from build123d import *

# Parameters (mm, degrees)
CROQUIS1_W              = 1660
CROQUIS1_H              = 810
CROQUIS1_W_2            = 300
CROQUIS1_H_2            = 5
SALIENTE_EXTRUIR3_DEPTH = 5
CROQUIS2_W              = 5
CROQUIS2_H              = 40
CROQUIS2_W_2            = 30
CROQUIS2_H_2            = 5
CROQUIS2_W_3            = 120
CROQUIS2_W_4            = 32.5
CROQUIS2_H_3            = 45
CROQUIS2_W_5            = 40
CORTAR_EXTRUIR2_DEPTH   = 10
CROQUIS3_R              = 3.2
CORTAR_EXTRUIR3_DEPTH   = 10
CORTAR_EXTRUIR5_DEPTH   = 10


with BuildPart() as part:
    # Croquis1 → Saliente-Extruir3 (new body)
    with BuildSketch(Plane(origin=(0, 0, 0), x_dir=(1, 0, 0), z_dir=(0, 1, 0))):
        with Locations((-1267.044657187, -398.10267676)):
            Rectangle(CROQUIS1_W, CROQUIS1_H)
        Polygon((-447.044657187, -95.60267676), (-447.044657187, -240.60267676), (-452.044657187, -240.60267676), (-452.044657187, -95.60267676), (-452.044657187, -90.60267676), (-447.044657187, -90.60267676), align=None, mode=Mode.SUBTRACT)
        with Locations((-782.044657187, -5.60267676)):
            Rectangle(CROQUIS1_W_2, CROQUIS1_H_2, mode=Mode.SUBTRACT)
        with Locations((-1267.044657187, -5.60267676)):
            Rectangle(CROQUIS1_W_2, CROQUIS1_H_2, mode=Mode.SUBTRACT)
        with Locations((-1752.044657187, -5.60267676)):
            Rectangle(CROQUIS1_W_2, CROQUIS1_H_2, mode=Mode.SUBTRACT)
        Polygon((-452.044657187, -328.10267676), (-452.044657187, -473.10267676), (-447.044657187, -473.10267676), (-447.044657187, -328.10267676), (-447.044657187, -323.10267676), (-452.044657187, -323.10267676), align=None, mode=Mode.SUBTRACT)
        Polygon((-452.044657187, -560.60267676), (-452.044657187, -705.60267676), (-447.044657187, -705.60267676), (-447.044657187, -560.60267676), (-447.044657187, -555.60267676), (-452.044657187, -555.60267676), align=None, mode=Mode.SUBTRACT)
        Polygon((-2087.044657187, -705.60267676), (-2082.044657187, -705.60267676), (-2082.044657187, -560.60267676), (-2082.044657187, -555.60267676), (-2087.044657187, -555.60267676), (-2087.044657187, -560.60267676), align=None, mode=Mode.SUBTRACT)
        Polygon((-2087.044657187, -473.10267676), (-2082.044657187, -473.10267676), (-2082.044657187, -328.10267676), (-2082.044657187, -323.10267676), (-2087.044657187, -323.10267676), (-2087.044657187, -328.10267676), align=None, mode=Mode.SUBTRACT)
        Polygon((-2087.044657187, -240.60267676), (-2082.044657187, -240.60267676), (-2082.044657187, -95.60267676), (-2082.044657187, -90.60267676), (-2087.044657187, -90.60267676), (-2087.044657187, -95.60267676), align=None, mode=Mode.SUBTRACT)
        with Locations((-1267.044657187, -790.60267676)):
            Rectangle(CROQUIS1_W_2, CROQUIS1_H_2, mode=Mode.SUBTRACT)
        with Locations((-782.044657187, -790.60267676)):
            Rectangle(CROQUIS1_W_2, CROQUIS1_H_2, mode=Mode.SUBTRACT)
        with Locations((-1752.044657187, -790.60267676)):
            Rectangle(CROQUIS1_W_2, CROQUIS1_H_2, mode=Mode.SUBTRACT)
    extrude(amount=SALIENTE_EXTRUIR3_DEPTH)

    # Croquis2 → Cortar-Extruir2 (cut)
    with BuildSketch(Plane(origin=(0, 5, 0), x_dir=(1, 0, 0), z_dir=(0, 1, 0))):
        with Locations((-1009.544657188, -443.10267676)):
            Rectangle(CROQUIS2_W, CROQUIS2_H)
        with Locations((-684.544657187, -635.60267676)):
            Rectangle(CROQUIS2_W_2, CROQUIS2_H_2)
        with Locations((-1127.044657187, -635.60267676)):
            Rectangle(CROQUIS2_W_3, CROQUIS2_H_2)
        with Locations((-1407.044657187, -635.60267676)):
            Rectangle(CROQUIS2_W_3, CROQUIS2_H_2)
        with Locations((-629.544657187, -635.60267676)):
            Rectangle(CROQUIS2_W_2, CROQUIS2_H_2)
        with Locations((-1404.544657188, -480.60267676)):
            Rectangle(CROQUIS2_W_3, CROQUIS2_H_2)
        with Locations((-785.794657187, -480.60267676)):
            Rectangle(CROQUIS2_W_4, CROQUIS2_H_2)
        with Locations((-833.294657187, -480.60267676)):
            Rectangle(CROQUIS2_W_4, CROQUIS2_H_2)
        with Locations((-604.544657187, -513.10267676)):
            Rectangle(CROQUIS2_W, CROQUIS2_H_3)
        with Locations((-864.544657187, -675.60267676)):
            Rectangle(CROQUIS2_W, CROQUIS2_H_3)
        with Locations((-1052.044657188, -315.60267676)):
            Rectangle(CROQUIS2_W_5, CROQUIS2_H_2)
        with Locations((-1142.044657188, -315.60267676)):
            Rectangle(CROQUIS2_W_5, CROQUIS2_H_2)
        with Locations((-1009.544657188, -353.10267676)):
            Rectangle(CROQUIS2_W, CROQUIS2_H)
        with Locations((-1124.544657188, -480.60267676)):
            Rectangle(CROQUIS2_W_3, CROQUIS2_H_2)
        with Locations((-604.544657187, -593.10267676)):
            Rectangle(CROQUIS2_W, CROQUIS2_H_3)
        with Locations((-1127.044657187, -160.60267676)):
            Rectangle(CROQUIS2_W_3, CROQUIS2_H_2)
        with Locations((-1407.044657187, -160.60267676)):
            Rectangle(CROQUIS2_W_3, CROQUIS2_H_2)
        with Locations((-864.544657187, -750.60267676)):
            Rectangle(CROQUIS2_W, CROQUIS2_H_3)
        with Locations((-1392.044657187, -315.60267676)):
            Rectangle(CROQUIS2_W_5, CROQUIS2_H_2)
        with Locations((-1929.544657187, -283.10267676)):
            Rectangle(CROQUIS2_W, CROQUIS2_H_3)
        with Locations((-1482.044657187, -315.60267676)):
            Rectangle(CROQUIS2_W_5, CROQUIS2_H_2)
        with Locations((-1700.794657187, -480.60267676)):
            Rectangle(CROQUIS2_W_4, CROQUIS2_H_2)
        with Locations((-1748.294657187, -480.60267676)):
            Rectangle(CROQUIS2_W_4, CROQUIS2_H_2)
        with Locations((-1929.544657187, -513.10267676)):
            Rectangle(CROQUIS2_W, CROQUIS2_H_3)
        with Locations((-1669.544657187, -750.60267676)):
            Rectangle(CROQUIS2_W, CROQUIS2_H_3)
        with Locations((-1524.544657187, -353.10267676)):
            Rectangle(CROQUIS2_W, CROQUIS2_H)
        with Locations((-1524.544657187, -443.10267676)):
            Rectangle(CROQUIS2_W, CROQUIS2_H)
        with Locations((-1669.544657187, -675.60267676)):
            Rectangle(CROQUIS2_W, CROQUIS2_H_3)
        with Locations((-1904.544657187, -635.60267676)):
            Rectangle(CROQUIS2_W_2, CROQUIS2_H_2)
        with Locations((-1929.544657187, -593.10267676)):
            Rectangle(CROQUIS2_W, CROQUIS2_H_3)
        with Locations((-1849.544657187, -635.60267676)):
            Rectangle(CROQUIS2_W_2, CROQUIS2_H_2)
        with Locations((-604.544657187, -283.10267676)):
            Rectangle(CROQUIS2_W, CROQUIS2_H_3)
        with Locations((-833.294657187, -315.60267676)):
            Rectangle(CROQUIS2_W_4, CROQUIS2_H_2)
        with Locations((-785.794657187, -315.60267676)):
            Rectangle(CROQUIS2_W_4, CROQUIS2_H_2)
        with Locations((-864.544657187, -45.60267676)):
            Rectangle(CROQUIS2_W, CROQUIS2_H_3)
        with Locations((-864.544657187, -120.60267676)):
            Rectangle(CROQUIS2_W, CROQUIS2_H_3)
        with Locations((-629.544657187, -160.60267676)):
            Rectangle(CROQUIS2_W_2, CROQUIS2_H_2)
        with Locations((-604.544657187, -203.10267676)):
            Rectangle(CROQUIS2_W, CROQUIS2_H_3)
        with Locations((-684.544657187, -160.60267676)):
            Rectangle(CROQUIS2_W_2, CROQUIS2_H_2)
        with Locations((-1849.544657187, -160.60267676)):
            Rectangle(CROQUIS2_W_2, CROQUIS2_H_2)
        with Locations((-1904.544657187, -160.60267676)):
            Rectangle(CROQUIS2_W_2, CROQUIS2_H_2)
        with Locations((-1669.544657187, -120.60267676)):
            Rectangle(CROQUIS2_W, CROQUIS2_H_3)
        with Locations((-1929.544657187, -203.10267676)):
            Rectangle(CROQUIS2_W, CROQUIS2_H_3)
        with Locations((-1669.544657187, -45.60267676)):
            Rectangle(CROQUIS2_W, CROQUIS2_H_3)
        with Locations((-1748.294657187, -315.60267676)):
            Rectangle(CROQUIS2_W_4, CROQUIS2_H_2)
        with Locations((-1700.794657187, -315.60267676)):
            Rectangle(CROQUIS2_W_4, CROQUIS2_H_2)
    extrude(amount=-CORTAR_EXTRUIR2_DEPTH, mode=Mode.SUBTRACT)

    # Croquis3 → Cortar-Extruir3 (cut)
    with BuildSketch(Plane(origin=(0, 5, 0), x_dir=(1, 0, 0), z_dir=(0, 1, 0))):
        with Locations(Location((-2084.544657187, -281.85267676, 0), (0, 0, 270))):
            Circle(CROQUIS3_R)
        with Locations(Location((-2084.544657187, -514.35267676, 0), (0, 0, 270))):
            Circle(CROQUIS3_R)
        with Locations(Location((-1509.544657187, -790.60267676, 0), (0, 0, 270))):
            Circle(CROQUIS3_R)
        with Locations(Location((-1024.544657187, -790.60267676, 0), (0, 0, 270))):
            Circle(CROQUIS3_R)
        with Locations(Location((-449.544657187, -514.35267676, 0), (0, 0, 270))):
            Circle(CROQUIS3_R)
        with Locations(Location((-449.544657187, -281.85267676, 0), (0, 0, 270))):
            Circle(CROQUIS3_R)
        with Locations(Location((-1024.544657187, -5.60267676, 0), (0, 0, 270))):
            Circle(CROQUIS3_R)
        with Locations(Location((-1509.544657187, -5.60267676, 0), (0, 0, 270))):
            Circle(CROQUIS3_R)
    extrude(amount=-CORTAR_EXTRUIR3_DEPTH, mode=Mode.SUBTRACT)

    # Croquis5 → Cortar-Extruir5 (cut)
    with BuildSketch(Plane(origin=(0, 5, 0), x_dir=(1, 0, 0), z_dir=(0, 1, 0))):
        Polygon((-1560.394657187, -177.84196813), (-1543.744657187, -177.84196813), (-1543.744657187, -160.34196813), (-1543.744657187, 6.89732324), (-2097.044657187, 6.89732324), (-2097.044657187, -803.10267676), (-437.044657187, -803.10267676), (-437.044657187, 6.89732324), (-990.344657187, 6.89732324), (-990.344657187, -160.34196813), (-990.344657187, -177.84196813), (-973.694657187, -177.84196813), (-973.694657187, -160.34196813), (-957.044657187, -160.34196813), (-957.044657187, -230.34196813), (-973.694657187, -230.34196813), (-973.694657187, -212.84196813), (-990.344657187, -212.84196813), (-990.344657187, -230.34196813), (-990.344657187, -398.10267676), (-1258.294657187, -398.10267676), (-1258.294657187, -390.60267676), (-1249.544657187, -390.60267676), (-1249.544657187, -383.10267676), (-1284.544657187, -383.10267676), (-1284.544657187, -390.60267676), (-1275.794657187, -390.60267676), (-1275.794657187, -398.10267676), (-1543.744657187, -398.10267676), (-1543.744657187, -230.34196813), (-1543.744657187, -212.84196813), (-1560.394657187, -212.84196813), (-1560.394657187, -230.34196813), (-1577.044657187, -230.34196813), (-1577.044657187, -160.34196813), (-1560.394657187, -160.34196813), align=None)
    extrude(amount=-CORTAR_EXTRUIR5_DEPTH, mode=Mode.SUBTRACT)


solid = part.part
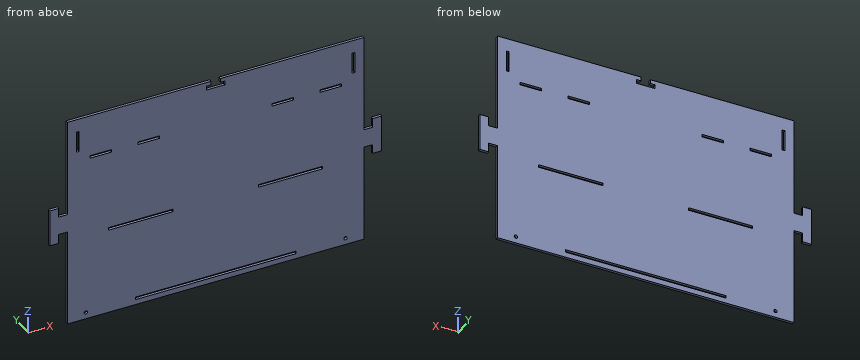
Read the model definition and answer for the solid it produces. Units are mm, in the model's axes. Give positions to 0.01 mm unless a question says otherwise; leave off trailing zeros. Write each loop counter-clockwise with the first axis right and the second up, starting at its lowest first coordinate (ties: lowest second). Pieces come first, ordered by that corner, then holes. Notation, with made-up numbers: (-15.5, 44.5) -> (0.5, 44.5) arc R21 ccw to (0.5, 79.5) -> close; hole circle Ø2 at (54, 57). An arc over 180 degrees is marked (long way). Answer as a JSON object with one key per item and string values. Group by question number.
1) Each of these flat-tipped pins is pushed along its axis until it touches: P1, Ø7.5, axis at x = -1024.54, z = 5.6, coming from the -Y side; P2, Ø1.5, axis at x = -982, y = 2, coming from the -Z side; P3, Ø2.5, axis at y = 1.5, z = 315, coming from the -X side. Where does it stop, or does it pass through?
2) Find section C-C (y = 1.65). Count the separate pieces of the cut face and the enclosed holes in it, and give its area (3 significant figures).
3) Find section B-B (z = 252). Write down the section's boundary in (x, y), and give its area (3 significant figures).
4) Consider L1, parallel to Z at x = -1126.5, y = 2.05; L2, parallel to X at y = 4.2, z = 372.5; L3, parallel to Z at x = -1010, y = 1.05. Determine where each line is inside the solid, lowest interval first. Write a range as from..to.
5) Find section A-A (x = -1405). Write down the section's boundary in (y, z).
Values follow:
{
 "1": {"P1": "stops at y = 0", "P2": "stops at z = 177.84", "P3": "stops at x = -1543.74"},
 "2": {"separate pieces": "1", "enclosed holes": "11", "area": "223,000 mm2"},
 "3": {"outline": "(-1543.74, 0) -> (-990.34, 0) -> (-990.34, 5) -> (-1543.74, 5) -> close", "area": "2,770 mm2"},
 "4": {"L1": "z = -6.9..3.1, 8.1..158.1, 163.1..313.1, 318.1..398.1", "L2": "x = -1543.74..-1527.04, -1522.04..-1012.04, -1007.04..-990.34", "L3": "z = -6.9..333.1, 373.1..398.1"},
 "5": {"outline": "(0, -6.9) -> (5, -6.9) -> (5, 3.1) -> (0, 3.1) -> close; (0, 8.1) -> (5, 8.1) -> (5, 158.1) -> (0, 158.1) -> close; (0, 163.1) -> (5, 163.1) -> (5, 313.1) -> (0, 313.1) -> close; (0, 318.1) -> (5, 318.1) -> (5, 398.1) -> (0, 398.1) -> close"}
}
